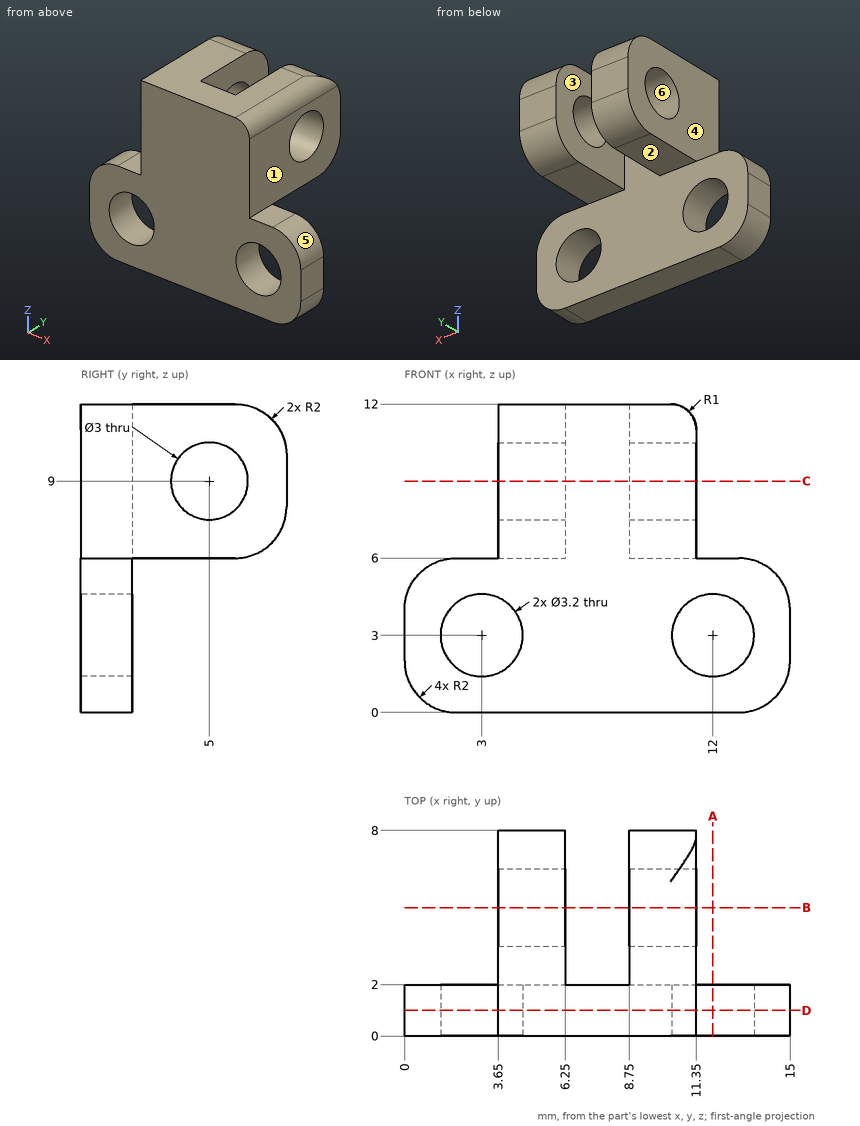
Check sheet for the drawn part. Datum: minimum x, y, z corner. Units: mm. A direction names the side the tool comes from. Give positions to 0.01 mm unless a question says otherwise; leave off trailing zeros. Write each loop counter-clockwise with the first axis right and the second up, starting at its lowest first coordinate (ties: lowest second). Pieces come first, ordered by that corner, then holes. Notation, with made-up numbers: (47.5, 46.25) -> (74.5, 46.25) arc R23 cw to (74.5, 85.25) -> close; hole circle Ø2 at (49.5, 74.25). An arc over 180 degrees is marked (long way). Use one line per item in the form item = value. Start each with the question number.
1. Mould release check, pull along Z, two halves, no side actions. Record for the marked faces 4, 5 and 6: pulls with the +Z half, pulls with the -Z half, needs draft (parallel to the pull), parting line crosses it, or undercut.
2. Access from +Z, -Z, +X, -X, +Y, -Y to the whole of each face (thin tool, end or side, straight path). Record for the marked faces 1, 2 and 3.
3. Section check A-A (x = 12). Record the cut outline in (y, z).
4. Section check D-D (y = 1). Record the cut outline in (x, z), and give its area (3 significant figures).
5. Go/stop test with flat-tipped pins: P1, Ø5, axis at x = 12, z = 3, coming from the +Y side; P2, Ø2, axis at x = 10, y = 3.5, coming from the -Z side; P3, Ø1.3, axis at x = 12.5, y = 0.5, coming from the +Z side. Record where each tip stops, or that it passes through.
6. Section check B-B (y = 5). Record the cut outline in (x, z), and give its area (3 significant figures).
7. Thickness scan on line 1 along X through (y, z) = (1.1, 3); line 2 along X through (y, z) = (6.5, 10); line 3 along Y through (x, z) = (5, 9). Record the ranges inside material, lowest first. Write a range as from..to.
8. Section check C-C (z = 9). Record the cut outline in (x, y).
Conclusion:
q1.face_4 = needs draft
q1.face_5 = pulls with the +Z half
q1.face_6 = undercut
q2.face_1 = +Z, +X, +Y, -Y
q2.face_2 = -Z, +X, -X, +Y
q2.face_3 = +Z, -Z, +Y
q3.outline = (0, 0) -> (2, 0) -> (2, 1.4) -> (0, 1.4) -> close; (0, 4.6) -> (2, 4.6) -> (2, 6) -> (0, 6) -> close
q4.outline = (0, 2) arc R2 ccw to (2, 0) -> (13, 0) arc R2 ccw to (15, 2) -> (15, 4) arc R2 ccw to (13, 6) -> (11.35, 6) -> (11.35, 11) arc R1 ccw to (10.35, 12) -> (3.65, 12) -> (3.65, 6) -> (2, 6) arc R2 ccw to (0, 4) -> close; hole circle Ø3.2 at (3, 3); hole circle Ø3.2 at (12, 3)
q4.area = 116 mm²
q5.P1 = 2
q5.P2 = 6
q5.P3 = 6
q6.outline = (3.65, 6) -> (6.25, 6) -> (6.25, 7.5) -> (3.65, 7.5) -> close; (3.65, 10.5) -> (6.25, 10.5) -> (6.25, 12) -> (3.65, 12) -> close; (8.75, 6) -> (11.35, 6) -> (11.35, 7.5) -> (8.75, 7.5) -> close; (8.75, 10.5) -> (11.35, 10.5) -> (11.35, 11) arc R1 ccw to (10.35, 12) -> (8.75, 12) -> close
q6.area = 15.4 mm²
q7.line_1 = 0..1.4, 4.6..10.4, 13.6..15
q7.line_2 = 3.65..6.25, 8.75..11.35
q7.line_3 = 0..3.5, 6.5..8
q8.outline = (3.65, 0) -> (11.35, 0) -> (11.35, 3.5) -> (8.75, 3.5) -> (8.75, 2) -> (6.25, 2) -> (6.25, 3.5) -> (3.65, 3.5) -> close; (3.65, 6.5) -> (6.25, 6.5) -> (6.25, 8) -> (3.65, 8) -> close; (8.75, 6.5) -> (11.35, 6.5) -> (11.35, 8) -> (8.75, 8) -> close
